```python
from build123d import *

# Parameters (mm, degrees)
SKETCH_1_W               = 384
SKETCH_1_H               = 604
RECESSED_TOP_SEAT_DEPTH  = 6
SKETCH_2_R               = 40
CENTRAL_ACCESS_DEPTH     = 716.756941985
SKETCH_3_R               = 3.5
FASTENER_CLEARANCE_DEPTH = 716.756941985
SKETCH_4_R               = 3.5
CUT_EXTRUDE_3_DEPTH      = 716.756941985
SKETCH_5_R               = 3.5
CUT_EXTRUDE_4_DEPTH      = 716.756941985
SKETCH_6_R               = 3.5
CUT_EXTRUDE_5_DEPTH      = 716.756941985


with BuildPart() as part:
    # 草图1 → Recessed_top_seat (new body)
    with BuildSketch(Plane.XY):
        with Locations((192, 302)):
            Rectangle(SKETCH_1_W, SKETCH_1_H)
    extrude(amount=RECESSED_TOP_SEAT_DEPTH)

    # 草图2 → Central_access (cut, through all)
    with BuildSketch(Plane.XY.offset(6)):
        with Locations((192, 302)):
            Circle(SKETCH_2_R)
    extrude(amount=-CENTRAL_ACCESS_DEPTH, mode=Mode.SUBTRACT)

    # 草图3 → Fastener_clearance (cut, through all)
    with BuildSketch(Plane.XY.offset(6)):
        with Locations((72, 122)):
            Circle(SKETCH_3_R)
    extrude(amount=-FASTENER_CLEARANCE_DEPTH, mode=Mode.SUBTRACT)

    # 草图4 → 切除-拉伸3 (cut, through all)
    with BuildSketch(Plane.XY.offset(6)):
        with Locations((72, 482)):
            Circle(SKETCH_4_R)
    extrude(amount=-CUT_EXTRUDE_3_DEPTH, mode=Mode.SUBTRACT)

    # 草图5 → 切除-拉伸4 (cut, through all)
    with BuildSketch(Plane.XY.offset(6)):
        with Locations((312, 122)):
            Circle(SKETCH_5_R)
    extrude(amount=-CUT_EXTRUDE_4_DEPTH, mode=Mode.SUBTRACT)

    # 草图6 → 切除-拉伸5 (cut, through all)
    with BuildSketch(Plane.XY.offset(6)):
        with Locations((312, 482)):
            Circle(SKETCH_6_R)
    extrude(amount=-CUT_EXTRUDE_5_DEPTH, mode=Mode.SUBTRACT)


solid = part.part
```
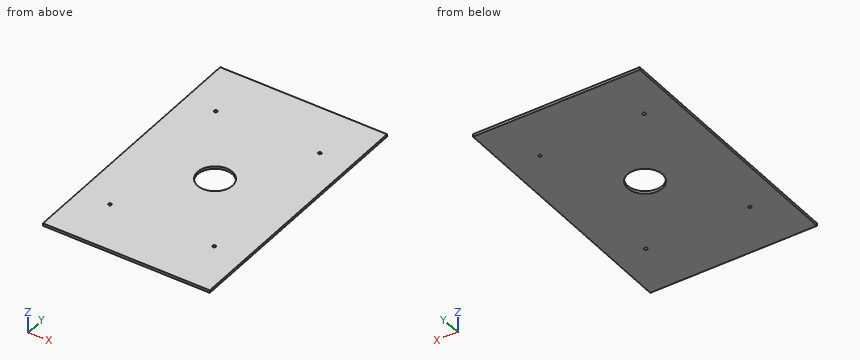
Here's how the part is built. I have some questions about the finished solid (model axes, mm). Round coordinates to 2 decimals unless told otherwise and drop trailing zeros. Write each loop counter-clockwise with the first axis right and the second up, starting at its lowest first coordinate (ties: lowest second). Pieces come first, ordered by that corner, then holes. Notation, with made-up numbers: M 12.5,6 L 35.5,6 A9 cw 35.5,23 Z; hole C 60.5,65.25 d3. An arc over 180 degrees is marked long. Answer as CSV lines item,"result". Start each with the question number.
1. Suppose I cut it at B-B on z = 2.95. Write out the boundary of the cut face in (x, y), then the cut area to 3 significant figures.
2. I need wall thicknesses on probe 1 along Y at (x, z) = (72, 3.45); probe 2 along X at (y, z) = (482, 1.75); probe 3 along Y at (x, z) = (313, 5.25). Which ranges of each line are inside material? Lowest first, please.
3. Suppose I cut it at A-A on x = 192. Write out the boundary of the cut face in (y, z), then the cut area to 3 significant figures.
4. Suppose I cut it at C-C on y = 322. Write out the boundary of the cut face in (x, z).
5. I'm going to push flat-ended pins straight in: pin 1 Ø6.5 at (x, y) = (312, 122) entering from +Z; pin 2 Ø4 at (x, y) = (333, 333.5) entering from -Z. Where does each tip first touch, or does it pass through?
Check result:
1,outline,"M 0,0 L 384,0 L 384,604 L 0,604 Z; hole C 72,122 d7; hole C 72,482 d7; hole C 192,302 d80; hole C 312,122 d7; hole C 312,482 d7"
1,area,"227,000 mm2"
2,probe 1,"y = 0 to 118.5, 125.5 to 478.5, 485.5 to 604"
2,probe 2,"x = 0 to 68.5, 75.5 to 308.5, 315.5 to 384"
2,probe 3,"y = 0 to 118.65, 125.35 to 478.65, 485.35 to 604"
3,outline,"M 0,0 L 262,0 L 262,6 L 0,6 Z; M 342,0 L 604,0 L 604,6 L 342,6 Z"
3,area,"3,140 mm2"
4,outline,"M 0,0 L 157.36,0 L 157.36,6 L 0,6 Z; M 226.64,0 L 384,0 L 384,6 L 226.64,6 Z"
5,pin 1,"passes through"
5,pin 2,"stops at z = 0"
